```python
from build123d import *

# Parameters (mm, degrees)
SKETCH_2_W               = 102
SKETCH_2_H               = 53.7
EXTRUDE_1_DEPTH          = 1.5
SKETCH_3_W               = 16.4
SKETCH_3_H               = 12.2
EXTRUDE_2_DEPTH          = 10.9
SKETCH_5_W               = 14
SKETCH_5_H               = 9
EXTRUDE_3_DEPTH          = 10.8
SKETCH_6_W               = 20.8
SKETCH_6_H               = 2.4
SKETCH_6_W_2             = 26.1
SKETCH_6_W_3             = 20.7
SKETCH_6_W_4             = 5
SKETCH_6_H_2             = 46.3
EXTRUDE_6_DEPTH          = 8.4
SKETCH_9_W               = 3.7
SKETCH_9_H               = 12
SKETCH_9_H_2             = 2.5
CUT_EXTRUDE_1_DEPTH      = 69.545367627
CHAMFER_1_SIZE           = 3.7
CUT_EXTRUDE_2_DEPTH      = 69.545367627
CUT_EXTRUDE_2_DEPTH_BACK = 69.545367627
SKETCH_7_R               = 1.65


with BuildPart() as part:
    # Эскиз2 → Бобышка-Вытянуть1 (new body)
    with BuildSketch(Plane(origin=(0, 0, 0), x_dir=(1, 0, 0), z_dir=(0, 1, 0))):
        with Locations((-2.938983051, 0.638135593)):
            Rectangle(SKETCH_2_W, SKETCH_2_H)
    extrude(amount=EXTRUDE_1_DEPTH)

    # Эскиз3 → Бобышка-Вытянуть2 (add)
    with BuildSketch(Plane(origin=(0, 1.5, 0), x_dir=(1, 0, 0), z_dir=(0, 1, 0))):
        with Locations((-53.638983051, 13.988135593)):
            Rectangle(SKETCH_3_W, SKETCH_3_H)
    extrude(amount=EXTRUDE_2_DEPTH)

    # Эскиз5 → Бобышка-Вытянуть3 (add)
    with BuildSketch(Plane(origin=(0, 1.5, 0), x_dir=(1, 0, 0), z_dir=(0, 1, 0))):
        with Locations((-52.038983051, -14.411864407)):
            Rectangle(SKETCH_5_W, SKETCH_5_H)
    extrude(amount=EXTRUDE_3_DEPTH)

    # Эскиз6 → Бобышка-Вытянуть6 (add)
    with BuildSketch(Plane(origin=(0, 1.5, 0), x_dir=(1, 0, 0), z_dir=(0, 1, 0))):
        with Locations((-16.838983051, -24.011864407)):
            Rectangle(SKETCH_6_W, SKETCH_6_H)
        with Locations((5.961016949, -24.011864407)):
            Rectangle(SKETCH_6_W, SKETCH_6_H)
        with Locations((28.761016949, -24.011864407)):
            Rectangle(SKETCH_6_W, SKETCH_6_H)
        with Locations((-23.088983051, 25.288135593)):
            Rectangle(SKETCH_6_W_2, SKETCH_6_H)
        with Locations((1.311016949, 25.288135593)):
            Rectangle(SKETCH_6_W_3, SKETCH_6_H)
        with Locations((24.061016949, 25.288135593)):
            Rectangle(SKETCH_6_W, SKETCH_6_H)
        with Locations((41.661016949, 3.088135593)):
            Rectangle(SKETCH_6_W_4, SKETCH_6_H_2)
    extrude(amount=EXTRUDE_6_DEPTH)

    # Эскиз9 → Вырез-Вытянуть1 (cut, through all)
    with BuildSketch(Plane(origin=(0, 1.5, 0), x_dir=(1, 0, 0), z_dir=(0, 1, 0))):
        with Locations((46.211016949, 21.488135593)):
            Rectangle(SKETCH_9_W, SKETCH_9_H)
        with Locations((46.211016949, -24.961864407)):
            Rectangle(SKETCH_9_W, SKETCH_9_H_2)
    extrude(amount=-CUT_EXTRUDE_1_DEPTH, mode=Mode.SUBTRACT)

    # Фаска1
    chamfer_1_edges = [part.edges().sort_by_distance(p)[0] for p in [
        (48.061016949, 0.75, 23.711864407),
        (48.061016949, 0.75, -15.488135593),
    ]]
    chamfer(chamfer_1_edges, length=CHAMFER_1_SIZE - 0.0001)  # a hair under: the kernel refuses the full size

    # Эскиз7 → Вырез-Вытянуть2 (cut, two sides: drawn at the far end of the back side and taken through both)
    with BuildSketch(Plane(origin=(0, 1.5, 0), x_dir=(1, 0, 0), z_dir=(0, 1, 0)).offset(-CUT_EXTRUDE_2_DEPTH_BACK)):
        with Locations(Location((-37.788983051, 24.738135593, 0), (0, 0, 270))):
            Circle(SKETCH_7_R)
        with Locations(Location((-39.588983051, -23.461864407, 0), (0, 0, 270))):
            Circle(SKETCH_7_R)
        with Locations(Location((12.411016949, 9.438135593, 0), (0, 0, 270))):
            Circle(SKETCH_7_R)
        with Locations(Location((12.411016949, -18.701864407, 0), (0, 0, 270))):
            Circle(SKETCH_7_R)
        with Locations(Location((36.551016949, 24.738135593, 0), (0, 0, 270))):
            Circle(SKETCH_7_R)
        with Locations(Location((40.711016949, -23.461864407, 0), (0, 0, 270))):
            Circle(SKETCH_7_R)
    extrude(amount=CUT_EXTRUDE_2_DEPTH + CUT_EXTRUDE_2_DEPTH_BACK, mode=Mode.SUBTRACT)


solid = part.part
```
Part model, mm, in its own coordinate system. A direction names the side the tool comes from. Round coordinates to 2 decimals unless told otherwise and drop trailing zeros. Loops run counter-clockwise (first coordinate to the right, second up) from the corner with the lowest first, then second, coordinate; pieces in that order, holes last.
Item 1: Cut at B-B, the plane z = 7. Give the cut face in (x, y), then the cut area to 3 significant figures.
Item 2: Drill centre lines: line 1 (X direction, y = 6.25, z = -18); line 2 (Z direction, x = -8, y = 3.5); line 3 (X direction, y = 7, z = 16.5). Where is each one in solid material? Low to high.
Item 3: Cut at D-D, the plane x = -50.5. Give the cut face in (y, z), then the cut area to 3 significant figures.
Item 4: 3-axis set-ups, long thin cutter, end or side, ignore diameter. For faces 1 (the face through (6, 6, 22.812)), 2 (the face through (-52, 12.3, 14)), 3 (the face through (-58, 1.5, -14)): which of +Z, -Z, +X, -X, +Y, -Y reach the whole face in a straight line?
Item 5: Mould opens along X. For faces 4 (the face through (46.185, 0.76, 21.888)), 5 (the face through (-4, 1.5, -1)), 6 (the face through (42, 6, 20.062)) say: +X half, -X half, draft (parallel to the pull), parting line (faces both ways), or undercut.
Item 6: Cut at A-A, the plane x = -33. Give the cut face in (y, z).
Item 7: Drop flat-ended pins along their axis: P1, Ø3, axis at x = -9, y = 6.5, coming from the +Z side; P2, Ø2.5, axis at y = 7.5, z = -25, coming from the -X side; P3, Ø10, axis at x = -50.5, z = 14.5, coming from the +Y side. Give the stop position or say it passes through.
Item 8: Cut at C-C, the plane y = 4. State how many separate pieces and enclosed holes the cut face has, then the cut area to 3 significant figures.
A:
1. outline: (-53.94, 0) - (48.06, 0) - (48.06, 1.5) - (44.16, 1.5) - (44.16, 9.9) - (39.16, 9.9) - (39.16, 1.5) - (-53.94, 1.5) - close
1. area: 195 mm2
2. line 1: x = -61.84 to -45.44, 39.16 to 44.16
2. line 2: z = -26.49 to -24.09, 22.81 to 25.21
2. line 3: x = -59.04 to -45.04, 39.16 to 44.16
3. outline: (0, -27.49) - (1.5, -27.49) - (1.5, -20.09) - (12.4, -20.09) - (12.4, -7.89) - (1.5, -7.89) - (1.5, 9.91) - (12.3, 9.91) - (12.3, 18.91) - (1.5, 18.91) - (1.5, 26.21) - (0, 26.21) - close
3. area: 311 mm2
4. face 1: +X, -X, +Y
4. face 2: +Z, +X, -X, +Y
4. face 3: +Z, -Z, -X, -Y
5. face 4: +X half
5. face 5: undercut
5. face 6: draft
6. outline: (0, -27.49) - (1.5, -27.49) - (1.5, -26.49) - (9.9, -26.49) - (9.9, -24.09) - (1.5, -24.09) - (1.5, 26.21) - (0, 26.21) - close
7. P1: stops at z = 25.21
7. P2: stops at x = -36.14
7. P3: stops at y = 12.3
8. separate pieces: 9
8. enclosed holes: 0
8. area: 870 mm2
